Here's the drawing with two shaded views (mm, measured from the low corner). I have some questions. A direction names the side the tool comes from. Give positions to 0.01 mm unless a question says otherwise; leave off trailing zeros. Loops run counter-clockwise (first coordinate to the right, second up) from the corner with the lowest first, then second, coordinate; pieces in that order, holes last. Notation, with made-up numbers: M -9,84.5 L 24,84.5 A31 cw 24,111.5 Z; hole C 73,17.5 d1. An arc over 180 degrees is marked long. Put each result on its own line as item: value. Start each with the question number.
1) Please list where these lines run through material, in increasing order: line 1 along Y through (x, z) = (11, 8); line 2 along Z through (x, y) = (30.5, 3.25); line 3 along X through (y, z) = (5.5, 3). Write a range as from..to.
2) Imagine slicing it at C-C (x = 27). Write out the boundary of the cut face in (y, z).
3) Imagine slicing it at B-B (z = 6.35). Write out the boundary of the cut face in (x, y).
4) For P1, Ø3, axis at y = 10.5, z = 5, coming from the -X side; P2, Ø3, axis at y = 3, z = 11, coming from the -X side; P3, Ø4.5, axis at y = 3, z = 2.5, coming from the -X side, each with a flat end and sliding along its axis, tell me the tip position at first contact or that it passes through.
5) Imagine slicing it at A-A (y = 5.5). Write out the boundary of the cut face in (x, z).
6) If we mould it in two halves opening along X, with no side actions, what happens to the marked faces 1, 2 and 3? For each: +X half, -X half, draft (parallel to the pull), parting line (faces both ways), or undercut.
7) Imagine slicing it at D-D (y = 8.5). Write out the boundary of the cut face in (x, z).
8) For the marked faces 4 and 5, which set-ups out of +Z, -Z, +X, -X, +Y, -Y let a thin tool reach every point of the face, with its end or its side?
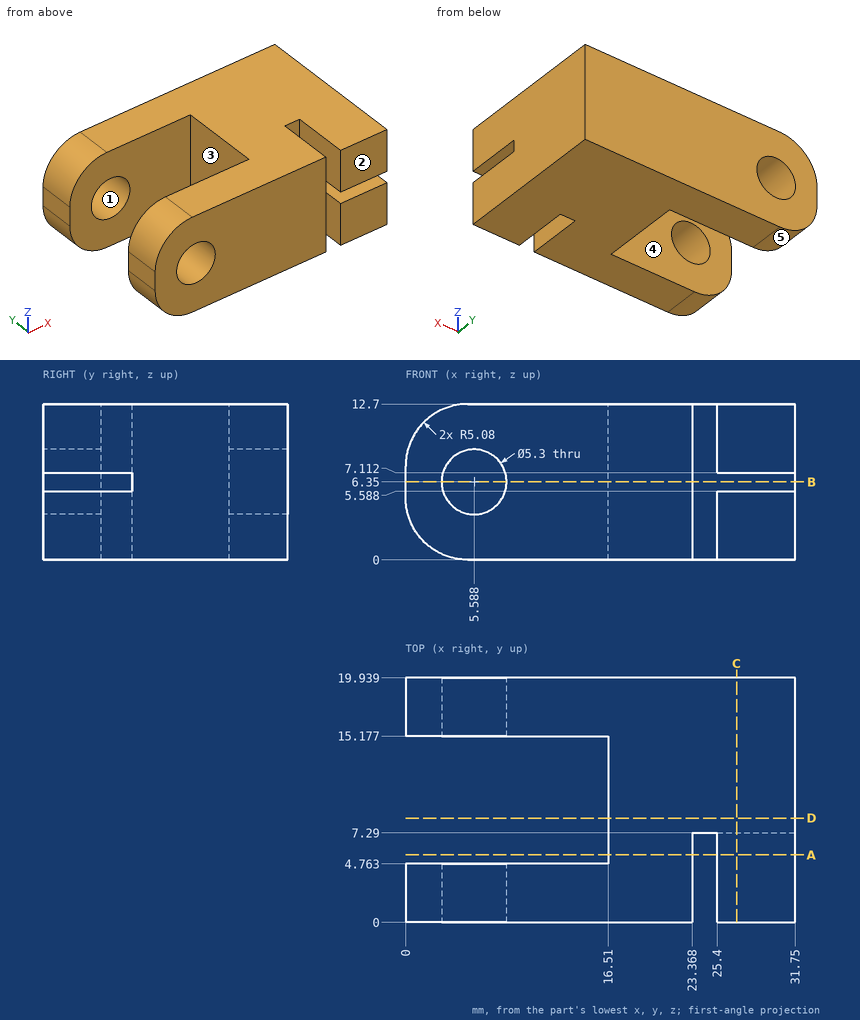
Recorded:
1. line 1: 0..4.76, 15.18..19.94
1. line 2: 0..5.59, 7.11..12.7
1. line 3: 16.51..23.37, 25.4..31.75
2. outline: M 0,0 L 19.94,0 L 19.94,12.7 L 0,12.7 L 0,7.11 L 7.29,7.11 L 7.29,5.59 L 0,5.59 Z
3. outline: M 0,0 L 2.94,0 L 2.94,4.76 L 0,4.76 Z; M 0,15.18 L 2.94,15.18 L 2.94,19.94 L 0,19.94 Z; M 8.24,0 L 23.37,0 L 23.37,7.29 L 31.75,7.29 L 31.75,19.94 L 8.24,19.94 L 8.24,15.18 L 16.51,15.18 L 16.51,4.76 L 8.24,4.76 Z
4. P1: x = 16.51
4. P2: x = 0.36
4. P3: x = 0.01
5. outline: M 16.51,0 L 23.37,0 L 23.37,12.7 L 16.51,12.7 Z; M 25.4,0 L 31.75,0 L 31.75,5.59 L 25.4,5.59 Z; M 25.4,7.11 L 31.75,7.11 L 31.75,12.7 L 25.4,12.7 Z
6. face 1: undercut
6. face 2: draft
6. face 3: -X half
7. outline: M 16.51,0 L 31.75,0 L 31.75,12.7 L 16.51,12.7 Z
8. face 4: +Z, -Z, -X
8. face 5: -Z, -X, +Y, -Y
